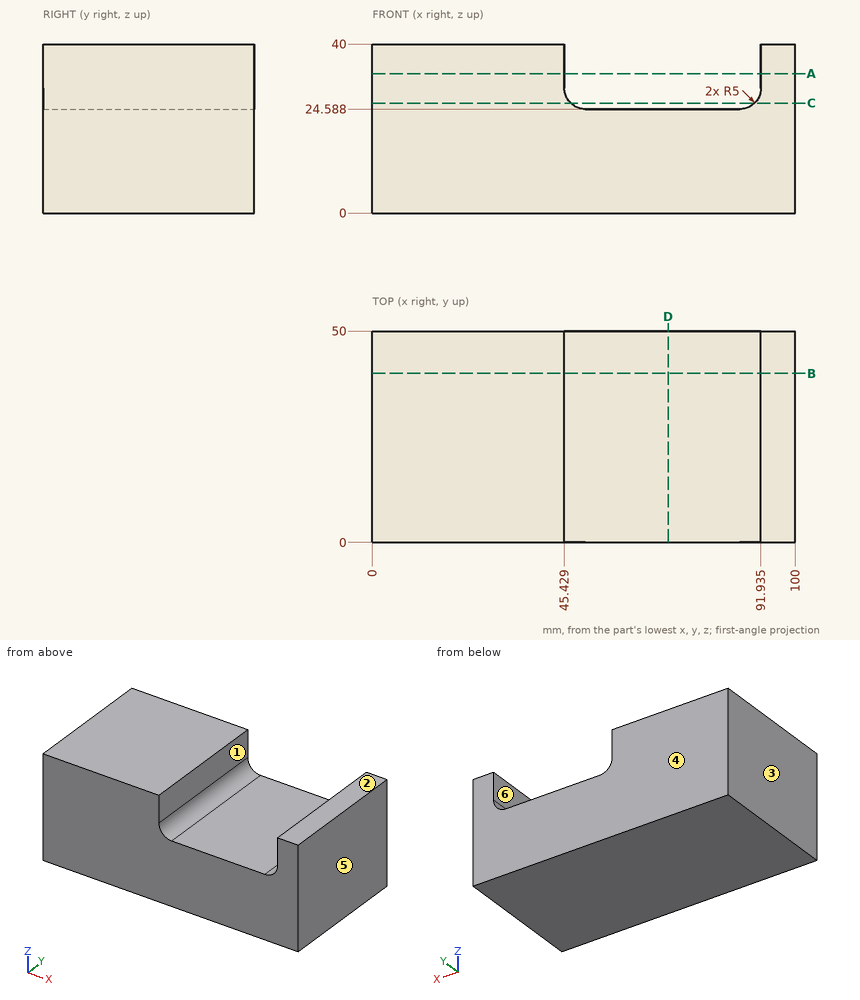
Print and shaded views of the part. All mm, measured from the part's lowest x, y and z. A direction names the side the tool comes from. Round coordinates to 2 decimals unless told otherwise and drop trailing zeros. Write each loop counter-clockwise with the first axis right and the second up, starting at its lowest first coordinate (ties: lowest second). Pieces come first, ordered by that corner, then holes. Notation, with made-up numbers: M -35.5,3.25 L -27.5,3.25 A11 cw -27.5,23.25 Z; hole C 82.5,3 d10. An arc over 180 degrees is marked long. One line per question, with ' | ' between items.
(1) Saw through at C-C on z = 26. Write the cut outline in (x, y), then the cut area to 3 significant figures.
Answer key:
outline: M 0,0 L 46.95,0 L 46.95,50 L 0,50 Z; M 90.42,0 L 100,0 L 100,50 L 90.42,50 Z | area: 2,830 mm^2
(2) Saw through at D-D on x = 70. Write the cut outline in (y, z).
Answer key:
outline: M 0,0 L 50,0 L 50,24.59 L 0,24.59 Z
(3) Pin check, flat tip, straight feed: pin 1 (11 mm diameter, centred on x = 65, y = 31.5, fed in from +Z). Stop position of the tip, or through.
Answer key:
pin 1: stops at z = 24.59
(4) Probe line 1 along X through (y, z) = (28, 35) (1 decimal); line 2 along Z through (x, y) = (66, 16.5); line 3 along X through (y, z) = (31, 26) (1 decimal). List the from-to ranges inside material, lowest first.
Answer key:
line 1: x = 0 to 45.4, 91.9 to 100 | line 2: z = 0 to 24.59 | line 3: x = 0 to 46.9, 90.4 to 100
(5) Two-plate mould, pull along X, no slides. Class the marked faces 3, 4, 5 and 6: released by +X, released by -X, zero draft, split by the parting line, or undercut.
Answer key:
face 3: released by -X | face 4: zero draft | face 5: released by +X | face 6: undercut
(6) Saw through at B-B on y = 40. Write the cut outline in (x, z) (1 decimal).
Answer key:
outline: M 0,0 L 100,0 L 100,40 L 91.9,40 L 91.9,29.6 A5 cw 86.9,24.6 L 50.4,24.6 A5 cw 45.4,29.6 L 45.4,40 L 0,40 Z
(7) 3-axis set-ups, long thin cutter, end or side, ignore diameter. For the marked faces 1 and 2: which of +Z, -Z, +X, -X, +Y, -Y reach the whole face in a straight line?
Answer key:
face 1: +Z, +Y, -Y | face 2: +Z, +X, -X, +Y, -Y
(8) Saw through at A-A on z = 33. Write the cut outline in (x, y) (1 decimal).
Answer key:
outline: M 0,0 L 45.4,0 L 45.4,50 L 0,50 Z; M 91.9,0 L 100,0 L 100,50 L 91.9,50 Z
